```python
from build123d import *

# Parameters (mm, degrees)
RESSALTO_EXTRUS_O1_DEPTH = 2
ESBO_O2_R                = 1.5
CORTE_EXTRUS_O1_DEPTH    = 10
CORTE_EXTRUS_O2_DEPTH    = 10


with BuildPart() as part:
    # Esboço1 → Ressalto-extrusão1 (new body)
    with BuildSketch(Plane(origin=(0, 0, 0), x_dir=(1, 0, 0), z_dir=(0, 1, 0))):
        with BuildLine():
            Line((-40.816022398, 183.1144834), (119.183977602, 183.1144834))
            ThreePointArc((119.183977602, 183.1144834), (133.326113225, 177.256619024), (139.183977602, 163.1144834))
            Line((139.183977602, 163.1144834), (139.183977602, 53.1144834))
            ThreePointArc((139.183977602, 53.1144834), (133.326113225, 38.972347776), (119.183977602, 33.1144834))
            Line((119.183977602, 33.1144834), (-40.816022398, 33.1144834))
            ThreePointArc((-40.816022398, 33.1144834), (-54.958158022, 38.972347776), (-60.816022398, 53.1144834))
            Line((-60.816022398, 53.1144834), (-60.816022398, 163.1144834))
            ThreePointArc((-60.816022398, 163.1144834), (-54.958158022, 177.256619024), (-40.816022398, 183.1144834))
        make_face()
    extrude(amount=RESSALTO_EXTRUS_O1_DEPTH)

    # Esboço2 → Corte-extrusão1 (cut)
    with BuildSketch(Plane(origin=(0, 2, 0), x_dir=(1, 0, 0), z_dir=(0, 1, 0))):
        with Locations(Location((1.183977602, 163.1144834, 0), (0, 0, 270))):
            Circle(ESBO_O2_R)
        with Locations(Location((77.183977602, 163.1144834, 0), (0, 0, 270))):
            Circle(ESBO_O2_R)
        with Locations(Location((77.183977602, 53.1144834, 0), (0, 0, 270))):
            Circle(ESBO_O2_R)
        with Locations(Location((1.183977602, 53.1144834, 0), (0, 0, 270))):
            Circle(ESBO_O2_R)
    extrude(amount=-CORTE_EXTRUS_O1_DEPTH, mode=Mode.SUBTRACT)

    # Esboço3 → Corte-extrusão2 (cut)
    with BuildSketch(Plane(origin=(0, 2, 0), x_dir=(1, 0, 0), z_dir=(0, 1, 0))):
        with BuildLine():
            Line((29.183977602, 141.1144834), (49.183977602, 141.1144834))
            ThreePointArc((49.183977602, 141.1144834), (56.255045413, 138.185551212), (59.183977602, 131.1144834))
            Line((59.183977602, 131.1144834), (59.183977602, 85.1144834))
            ThreePointArc((59.183977602, 85.1144834), (56.255045413, 78.043415588), (49.183977602, 75.1144834))
            Line((49.183977602, 75.1144834), (29.183977602, 75.1144834))
            ThreePointArc((29.183977602, 75.1144834), (22.11290979, 78.043415588), (19.183977602, 85.1144834))
            Line((19.183977602, 85.1144834), (19.183977602, 131.1144834))
            ThreePointArc((19.183977602, 131.1144834), (22.11290979, 138.185551212), (29.183977602, 141.1144834))
        make_face()
    extrude(amount=-CORTE_EXTRUS_O2_DEPTH, mode=Mode.SUBTRACT)


solid = part.part
```
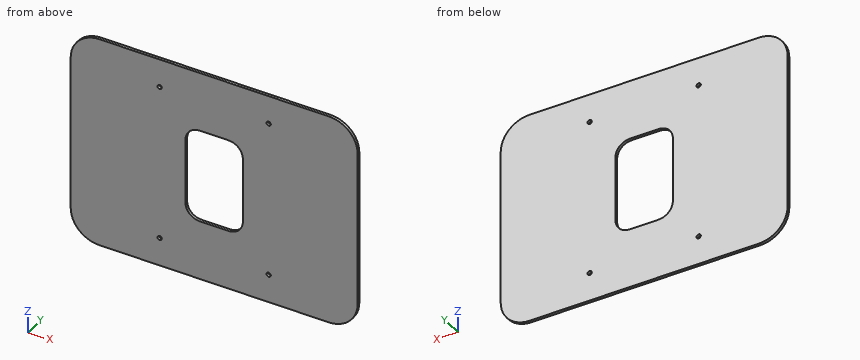
Check sheet for the modelled part. Datum: model origin and axes. Units: mm. Coordinates: 2 decimals unless noted, no trailing zeros. Loops run counter-clockwise (first coordinate to the right, second up) from the corner with the lowest first, then second, coordinate; pieces in that order, holes last. Notation, with made-up numbers: M 69,54.5 L 128,54.5 A25 ccw 128,89.5 Z; hole C 85.5,-37 d9. An arc over 180 degrees is marked long. Answer as a JSON object with one key per item and string values.
1. Sectioned sample at B-B on x = 23. Record the cut outline in (y, z), and give its area (3 significant figures).
Outcome:
{"outline": "M 0,-183.11 L 2,-183.11 L 2,-138.97 L 0,-138.97 Z; M 0,-77.26 L 2,-77.26 L 2,-33.11 L 0,-33.11 Z", "area": "177 mm²"}
2. Sectioned sample at D-D on z = -44. Record the cut outline in (x, y).
Outcome:
{"outline": "M -58.62,0 L 136.99,0 L 136.99,2 L -58.62,2 Z"}
3. Depth check by flat-ended pin: P1, Ø5, axis at x = -5, z = -48.5, coming from the -Y side. Enter the tip coordinate at first touch or a pass-through.
Outcome:
{"P1": "y = 0"}
4. Sectioned sample at C-C on y = 0.4. Record the cut outline in (x, z), and give its area (3 significant figures).
Outcome:
{"outline": "M -60.82,-163.11 A20 ccw -40.82,-183.11 L 119.18,-183.11 A20 ccw 139.18,-163.11 L 139.18,-53.11 A20 ccw 119.18,-33.11 L -40.82,-33.11 A20 ccw -60.82,-53.11 Z; hole C 1.18,-163.11 d3; hole C 1.18,-53.11 d3; hole M 19.18,-131.11 A10 ccw 29.18,-141.11 L 49.18,-141.11 A10 ccw 59.18,-131.11 L 59.18,-85.11 A10 ccw 49.18,-75.11 L 29.18,-75.11 A10 ccw 19.18,-85.11 Z; hole C 77.18,-163.11 d3; hole C 77.18,-53.11 d3", "area": "27,100 mm²"}
5. Scan lines: L1, parallel to X at y = 1.4, z = -163; L2, parallel to Z at x = 36, y = 1.6; L3, parallel to X at y = 0.75, z = -103. Record each from-to range of solid material in increasing order. Write a range as from..to.
Outcome:
{"L1": "-60.82..-0.31, 2.68..75.69, 78.68..139.18", "L2": "-183.11..-141.11, -75.11..-33.11", "L3": "-60.82..19.18, 59.18..139.18"}
6. Sectioned sample at A-A on z = -121. Record the cut outline in (x, y), and give its area (3 significant figures).
Outcome:
{"outline": "M -60.82,0 L 19.18,0 L 19.18,2 L -60.82,2 Z; M 59.18,0 L 139.18,0 L 139.18,2 L 59.18,2 Z", "area": "320 mm²"}
